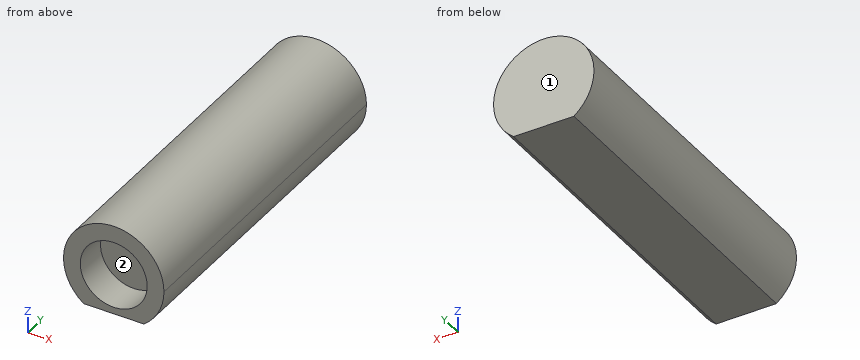
from build123d import *

# Parameters (mm, degrees)
F0_R     = 2.54
F1_DEPTH = 25.4
F2_DEPTH = 22.86


with BuildPart() as f1:
    # F0 (on Front) → F1 (new body)
    with BuildSketch(Plane.XZ):
        with BuildLine():
            ThreePointArc((2.286, -3.048), (3.407768, -1.703884), (3.81, 0))
            ThreePointArc((3.81, 0), (-1.703884, 3.407768), (-2.286, -3.048))
            Line((-2.286, -3.048), (2.286, -3.048))
        make_face()
        Circle(F0_R, mode=Mode.SUBTRACT)
    extrude(amount=F1_DEPTH)

    # F0 (on Front) → F2 (join)
    with BuildSketch(Plane.XZ):
        Circle(F0_R)
    extrude(amount=F2_DEPTH)


solid = f1.part
Input: part model. Units: mm. Frame: model coordinates. Face numbers are marked on the shaded views. A direction names the side the tool comes from. Give positions to 0.01 mm unless a question says otherwise; leave off trailing zeros. Write each loop counter-clockwise with the first axis right and the second up, starting at its lowest first coordinate (ties: lowest second). Pieces come first, ordered by that corner, then holes. Notation, with made-up numbers: M 13,20.25 L 46,20.25 A22 cw 46,54.25 Z; hole C 66,-38.75 d6. An arc over 180 degrees is marked long. Use one line per item in the form item = value.
1. Cut plane C-C on y = -17.25. Return loops of the section in (x, z).
Outcome:
outline = M -2.29,-3.05 L 2.29,-3.05 A3.81 ccw 3.81,0 A3.81 ccw long Z
2. Cut plane A-A on x = 0. Return loops of the section in (y, z), and give its area (3 significant figures).
Outcome:
outline = M -25.4,-3.05 L 0,-3.05 L 0,3.81 L -25.4,3.81 L -25.4,2.54 L -22.86,2.54 L -22.86,-2.54 L -25.4,-2.54 Z
area = 161 mm²
3. Cut plane B-B on z = 1.5. Return loops of the section in (x, y).
Outcome:
outline = M -3.5,-25.4 L -2.05,-25.4 L -2.05,-22.86 L 2.05,-22.86 L 2.05,-25.4 L 3.5,-25.4 L 3.5,0 L -3.5,0 Z
4. First-contact query: P1, Ø1.5, axis at y = -9.5, z = -1, coming from the +X side; P2, Ø1.5, axis at y = -13.5, z = 2, coming from the +X side; P3, Ø2, axis at y = -7.5, z = -1.5, coming from the -X side. Flat tips, straight axial feed; report the tip coordinate or a pass-through.
Outcome:
P1 = 3.8
P2 = 3.6
P3 = -3.78
5. Ray query, L1, parallel to Z at x = 0, y = -24.7; L2, parallel to Y at x = -1, z = 1; L3, parallel to X at y = -23.5, z = -1.5. Return the intervals inside material, ascending.
Outcome:
L1 = -3.05 to -2.54, 2.54 to 3.81
L2 = -22.86 to 0
L3 = -3.5 to -2.05, 2.05 to 3.5
6. Cut plane D-D on x = 3. Return loops of the section in (y, z), and give its area (3 significant figures).
Outcome:
outline = M -25.4,-2.35 L 0,-2.35 L 0,2.35 L -25.4,2.35 Z
area = 119 mm²
7. Reachability of the marked faces 1 and 2 from +Z, -Z, +X, -X, +Y, -Y: full face, straight path, thin tool, end or side. Return the list, or none.
Outcome:
face_1 = +Z, -Z, +X, -X, +Y
face_2 = -Y
